Verification items for the finished model (mm, model axes). Face numbers are marked on the shaded views. A direction names the side the tool comes from. Give positions to 0.01 mm unless a question says otherwise; leave off trailing zeros. Write each loop counter-clockwise with the first axis right and the second up, starting at its lowest first coordinate (ties: lowest second). Pieces come first, ordered by that corner, then holes. Notation, with made-up numbers: (85, 62) - (123, 62) arc R18 cw to (123, 78) - close; hole circle Ø8 at (81.5, 43.25). An arc over 180 degrees is marked (long way). Answer as a JSON object with one key per item and string values. Group by question number.
Item 1: Sectioned sample at A-A, the plane z = 4. Record the boundary of the cut face in (x, y).
Item 2: Sectioned sample at D-D, the plane y = -14. Record the boundary of the cut face in (x, z).
Item 3: Tool access check on the marked faces 1, 2 and 3. Record the directions out of +Z, -Z, +X, -X, +Y, -Y that give a thin tool (end or side, any length) a straight path to the whole face; none if there is none.
Item 4: Sectioned sample at B-B, the plane x = 6.75. Record the boundary of the cut face in (y, z), and give its area (3 significant figures).
Item 5: Scan lines: line 1 along Z through (x, y) = (-8.25, 0); line 2 along Z through (x, y) = (5.75, 16.5); line 3 along X through (y, z) = (13, 3.75). Record each from-to range of solid material in increasing order. Write a range as [from, to].
Item 6: Draft check along X on the marked faces 4, 5 and 6. Enter one of: +X half, -X half, draft (parallel to the pull), parting line (faces both ways), or undercut.
Item 7: Sectioned sample at C-C, the plane z = 25. Record the boundary of the cut face in (x, y).
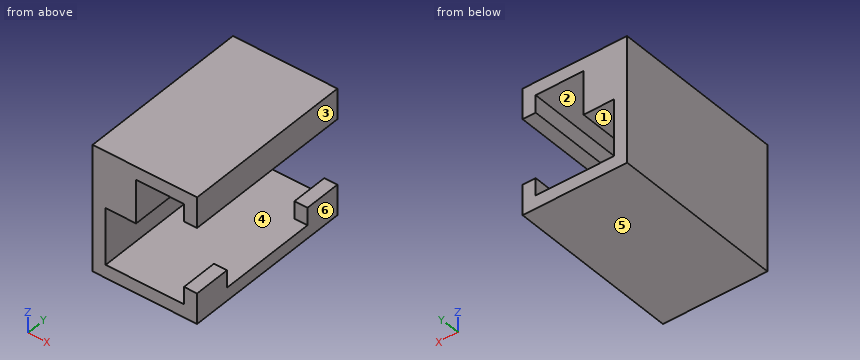
```python
from build123d import *

# Parameters (mm, degrees)
F0_W     = 24
F0_H     = 40
F1_DEPTH = 29
F2_W     = 18
F2_H     = 23
F3_DEPTH = 61.722
F4_W     = 3
F4_H     = 15
F5_DEPTH = 55.626
F6_W     = 23
F6_H     = 4
F7_DEPTH = 5.334
F8_W     = 7
F8_H     = 10
F9_DEPTH = 40


with BuildPart() as f1:
    # F0 (on Top) → F1 (new body)
    with BuildSketch(Plane.XY):
        Rectangle(F0_W, F0_H)
    extrude(amount=F1_DEPTH)

    # F2 (on face) → F3 (cut)
    with BuildSketch(Plane.XZ.offset(20)):
        with Locations((0, 14.5)):
            Rectangle(F2_W, F2_H)
    extrude(amount=-F3_DEPTH, mode=Mode.SUBTRACT)

    # F4 (on face) → F5 (cut)
    with BuildSketch(Plane.XZ.offset(20)):
        with Locations((10.5, 14.5)):
            Rectangle(F4_W, F4_H)
    extrude(amount=-F5_DEPTH, mode=Mode.SUBTRACT)

    # F6 (on face) → F7 (cut)
    with BuildSketch(Plane.YZ.offset(12)):
        with Locations((0, 5)):
            Rectangle(F6_W, F6_H)
    extrude(amount=-F7_DEPTH, mode=Mode.SUBTRACT)

    # F8 (on face) → F9 (join)
    with BuildSketch(Plane.XZ.offset(20)):
        with Locations((-5.5, 21)):
            Rectangle(F8_W, F8_H)
    extrude(amount=-F9_DEPTH)


solid = f1.part
```
Geometry check:
{
 "1": {"outline": "(-12, -20) - (-9, -20) - (-9, 20) - (-12, 20) - close; (9, -20) - (12, -20) - (12, -11.5) - (9, -11.5) - close; (9, 11.5) - (12, 11.5) - (12, 20) - (9, 20) - close"},
 "2": {"outline": "(-12, 0) - (12, 0) - (12, 7) - (9, 7) - (9, 3) - (-9, 3) - (-9, 16) - (-2, 16) - (-2, 26) - (9, 26) - (9, 22) - (12, 22) - (12, 29) - (-12, 29) - close"},
 "3": {"face 1": "+X, +Y, -Y", "face 2": "+Y, -Y", "face 3": "+Z, -Z, +X, +Y, -Y"},
 "4": {"outline": "(-20, 0) - (20, 0) - (20, 3) - (-20, 3) - close; (-20, 26) - (20, 26) - (20, 29) - (-20, 29) - close", "area": "240 mm^2"},
 "5": {"line 1": "[0, 3], [16, 29]", "line 2": "[0, 3], [26, 29]", "line 3": "[-12, -9], [9, 12]"},
 "6": {"face 4": "undercut", "face 5": "draft", "face 6": "+X half"},
 "7": {"outline": "(-12, -20) - (-2, -20) - (-2, 20) - (-12, 20) - close; (9, -20) - (12, -20) - (12, 20) - (9, 20) - close"}
}
